Source: CAD feature listing. Evaluate the final solid. Frame: model axes, mm. A direction names the side the tool comes from. Give positions to 0.01 mm unless a question says otherwise; leave off trailing zeros. Return JSON: item names as keys, results as strings. Group by question number.
(1) Ray query, line 1 (X direction, y = -2.5, z = -35); line 2 (X direction, y = -3.25, z = 30.5); line 3 (X direction, y = -1.3, z = 46). Return the intervals inside material, ascending. Write a range as from..to.
(2) Access query for faces 4 (the face through (-34, -2, 22.888)), 5 (the face through (0, -2, 27.821)), 6 (the face through (32, -2, 33.346)). Directions: +Z, -Z, +X, -X, +Y, -Y. A direction counts if a zero-diameter tool reaches every point of the face in a straight line with its end or side. Return the directions, or none.
(3) Pin query (flat end, axial travel): pin 1 (1.5 mm diameter, centred on y = -2.5, z = 34.5, fed in from +X); pin 2 (1.7 mm diameter, centred on y = -1.5, z = 13, fed in from +X). Return the tip coordinate at first contact, or that it passes through.
(4) Cut plane A-A on x = 45.5. Give the number of separate pieces and of enclosed holes in the cut face, then the cut area to 3 significant figures.
(5) Draft query along Z for faces 1 (the face through (-7.694, -1.726, 13.047)), 2 (the face through (0, -2, -31.227)), 3 (the face through (56.842, -2, 30)). Return one class per face: released by +Z, released by -Z, zero draft, split by the parting line, or undercut.
```python
from build123d import *

# Parameters (mm, degrees)
F0_W     = 71.032305
F0_H     = 3.316156
F0_W_2   = 70.65738
F0_H_2   = 4.029283
F0_W_3   = 70.945185
F0_H_3   = 4.029279
F0_W_4   = 71.23299
F0_H_4   = 3.453669
F0_W_5   = 71.426928
F0_H_5   = 3.551615
F0_W_6   = 72.216179
F0_H_6   = 3.354305
F0_W_7   = 72.610803
F0_H_7   = 2.762366
F0_W_8   = 73.005423
F0_H_8   = 3.354303
F0_W_9   = 72.808113
F0_H_9   = 3.354299
F1_DEPTH = 3.5


with BuildPart() as f1:
    # F0 (on Front) → F1 (new body)
    with BuildSketch(Plane.XZ):
        Polygon((56.841634, 59.431892), (-61.265364, 59.431892), (-61.265364, 47.354873), (-8.385758, 47.354873), (-8.385758, 44.197883), (-61.265364, 44.197883), (-61.265364, 36.305401), (-8.385758, 36.305401), (-8.385758, 33.345722), (-61.265364, 33.345722), (-61.265364, 25.847867), (-7.991134, 25.847867), (-7.991134, 22.888189), (-61.265364, 22.888189), (-61.265364, 14.798397), (-7.596511, 14.798397), (-7.793822, 11.246782), (-61.265364, 11.246782), (-61.265364, 3.597572), (-8.202464, 3.597572), (-8.202464, 0), (-61.265364, 0), (-61.265364, -9.641493), (-7.914659, -9.641493), (-7.914659, -13.382968), (-61.265364, -13.382968), (-61.265364, -24.031783), (-7.914659, -24.031783), (-7.914659, -27.485449), (-61.265364, -27.485449), (-61.265364, -38.134262), (-8.202464, -38.134262), (-8.202464, -42.163543), (-61.265364, -42.163543), (-61.265364, -53.076919), (-8.202464, -53.076919), (-8.202464, -55.690415), (-61.265364, -55.690415), (-61.265364, -69.217287), (56.841634, -69.217287), (56.841634, -56.036595), (11.206436, -56.036595), (11.206436, -53.076919), (56.841634, -53.076919), (56.841634, -42.163543), (11.206436, -42.163543), (11.080521, -38.134262), (56.841634, -38.134262), (56.841634, -28.348867), (6.475631, -28.348867), (6.475631, -24.031783), (56.841634, -24.031783), (56.841634, -13.382968), (6.475631, -13.382968), (6.475631, -9.641493), (56.841634, -9.641493), (56.841634, 0), (6.763437, 0), (6.475631, 3.597572), (56.841634, 3.597572), (56.841634, 11.444095), (6.412639, 11.444095), (6.412639, 14.798397), (56.841634, 14.798397), (56.841634, 22.690875), (6.215328, 22.690875), (6.215328, 25.847867), (56.841634, 25.847867), (56.841634, 33.345722), (6.215328, 33.345722), (6.215328, 36.305401), (56.841634, 36.305401), (56.841634, 44.000566), (6.018014, 44.000566), (6.018014, 47.354873), (56.841634, 47.354873), align=None)
        with Locations((0.690593, -47.27529)):
            Rectangle(F0_W, F0_H, mode=Mode.SUBTRACT)
        with Locations((0.50313, -33.241566)):
            Rectangle(F0_W_2, F0_H_2, mode=Mode.SUBTRACT)
        with Locations((0.647033, -19.714693)):
            Rectangle(F0_W_3, F0_H_3, mode=Mode.SUBTRACT)
        with Locations((0.790935, -4.173183)):
            Rectangle(F0_W_4, F0_H_4, mode=Mode.SUBTRACT)
        with Locations((0.887904, 7.695167)):
            Rectangle(F0_W_5, F0_H_5, mode=Mode.SUBTRACT)
        with Locations((0.690593, 18.448668)):
            Rectangle(F0_W_6, F0_H_6, mode=Mode.SUBTRACT)
        with Locations((0.887905, 29.202171)):
            Rectangle(F0_W_7, F0_H_7, mode=Mode.SUBTRACT)
        with Locations((1.085214, 40.350296)):
            Rectangle(F0_W_8, F0_H_8, mode=Mode.SUBTRACT)
        with Locations((0.98656, 51.202455)):
            Rectangle(F0_W_9, F0_H_9, mode=Mode.SUBTRACT)
    extrude(amount=F1_DEPTH)


solid = f1.part
```
Answers:
{
 "1": {"line 1": "-61.27..-34.83, 35.83..56.84", "line 2": "-61.27..-35.42, 37.19..56.84", "line 3": "-8.39..6.02"},
 "2": {"face 4": "-X, +Y, -Y", "face 5": "+Y, -Y", "face 6": "+X, +Y, -Y"},
 "3": {"pin 1": "x = 6.22", "pin 2": "x = 6.41"},
 "4": {"separate pieces": "10", "enclosed holes": "0", "area": "340 mm²"},
 "5": {"face 1": "undercut", "face 2": "undercut", "face 3": "zero draft"}
}
